Input: dimensioned drawing with shaded views. Units: mm. Origin: part minimum x, y, z. Give positions to 0.01 mm unless a question says otherwise; leave off trailing zeros. Order: outer loops, then holes, each group sorted by start corner. A loop starts at its lowest first (then second) coordinate and runs counter-clockwise, first axis right, second up. Notation, with made-up numbers: (-12, 42.25) - (38, 42.25) arc R29 cw to (38, 71.25) - close; hole circle Ø1 at (43, -25.5). An arc over 180 degrees is marked (long way). Use a Markdown table: item, result.
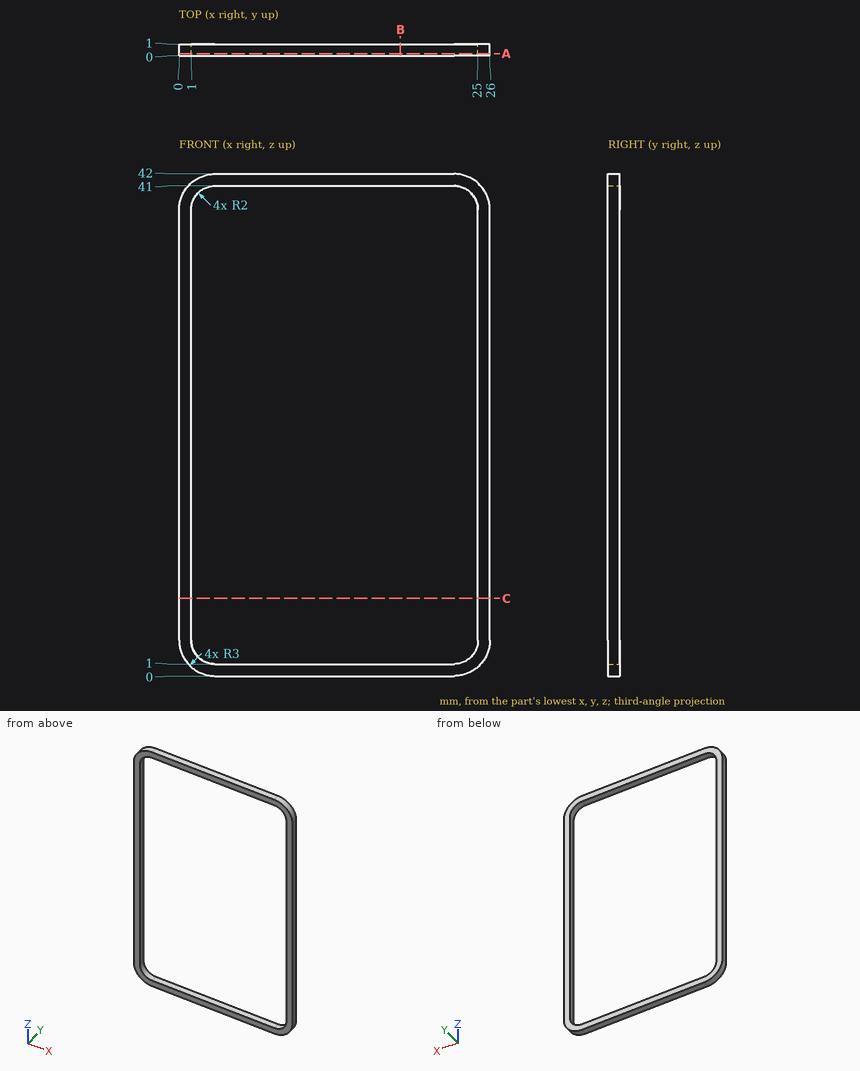
1. Material intervals for line 1 along X through (y, z) = (0.75, 10.5); line 2 along Z through (x, y) = (12, 0.6), sorted ascending.
Response:
| item | result |
|---|---|
| line 1 | x = 0 to 1, 25 to 26 |
| line 2 | z = 0 to 1, 41 to 42 |
2. Section query B-B (x = 18.5). Return loops of the section in (y, z), then the cut area to 3 significant figures.
Response:
| item | result |
|---|---|
| outline | (0, 0) - (1, 0) - (1, 1) - (0, 1) - close; (0, 41) - (1, 41) - (1, 42) - (0, 42) - close |
| area | 2.00 mm^2 |
3. Section query A-A (y = 0.2). Return loops of the section in (x, z).
Response:
| item | result |
|---|---|
| outline | (0, 3) arc R3 ccw to (3, 0) - (23, 0) arc R3 ccw to (26, 3) - (26, 39) arc R3 ccw to (23, 42) - (3, 42) arc R3 ccw to (0, 39) - close; hole (1, 3) arc R2 ccw to (3, 1) - (23, 1) arc R2 ccw to (25, 3) - (25, 39) arc R2 ccw to (23, 41) - (3, 41) arc R2 ccw to (1, 39) - close |
4. Section query C-C (z = 6.5). Return loops of the section in (x, y), then the cut area to 3 significant figures.
Response:
| item | result |
|---|---|
| outline | (0, 0) - (1, 0) - (1, 1) - (0, 1) - close; (25, 0) - (26, 0) - (26, 1) - (25, 1) - close |
| area | 2.00 mm^2 |
